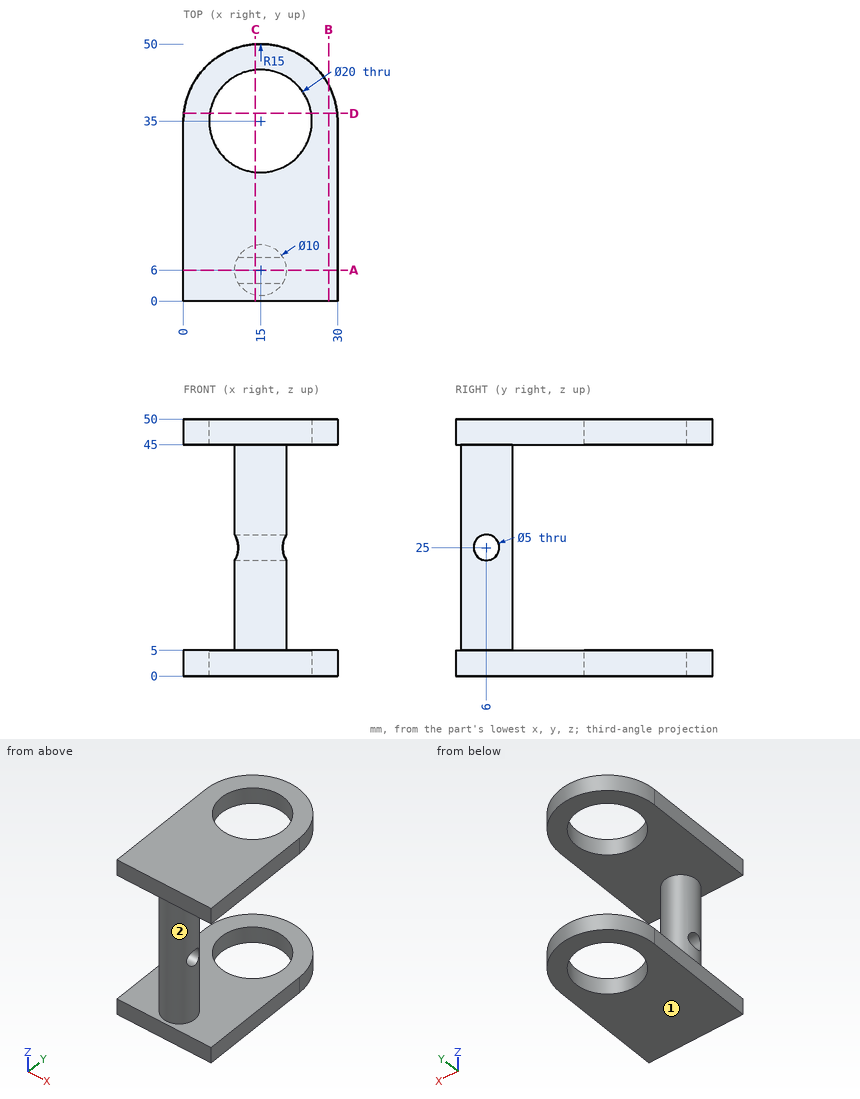
For this review, use the dimensioned drawing (mm, ordinates from the lowest corner) and the shaded views. A direction names the side the tool comes from. Give positions to 0.01 mm unless a question says otherwise; leave off trailing zeros. Order: outer loops, then holes, each group sorted by start corner. A loop starts at its lowest first (then second) coordinate and runs counter-clockwise, first axis right, second up.
1) Wall thickness on line 1 (Z direction, x = 9.75, y = 10.5); line 2 (Y direction, x = 15, z = 3.1); line 3 (Z direction, x = 15.5, y = 6): over which ranges is each line inside the solid? List them lowest first.
2) Take a section at D-D (y = 36.5). Give the boundary of the cut face in (x, z), then the cut area to 3 significant figures.
3) Take a section at B-B (x = 28.25). Give the boundary of the cut face in (y, z).
4) Take a section at A-A (y = 6). Give the boundary of the cut face in (x, z).
5) Take a section at C-C (x = 14). Give the boundary of the cut face in (y, z).
6) Insertion check: pin 1 (9 mm diameter, centred on x = 13.5, y = 12.5, fed in from -Z); pin 2 (4 mm diameter, centred on y = 6, z = 25, fed in from +X); pin 3 (6 mm diameter, centred on x = 15, z = 15.5, fed in from -Y). Each pin has a flat end and moves straight along its axis. Give the tip position at first contact, or say it passes through.
7) For the marked faces 1 and 2, list the 3-axis set-ups (+Z, -Z, +X, -X, +Y, -Y) from which the entire face can be reached by the end or side of a thin tool; tool diameter is ignored.
Derived:
1. line 1: z = 0 to 5, 45 to 50
1. line 2: y = 0 to 25, 45 to 50
1. line 3: z = 0 to 22.5, 27.5 to 50
2. outline: (0.08, 0) - (5.11, 0) - (5.11, 5) - (0.08, 5) - close; (0.08, 45) - (5.11, 45) - (5.11, 50) - (0.08, 50) - close; (24.89, 0) - (29.92, 0) - (29.92, 5) - (24.89, 5) - close; (24.89, 45) - (29.92, 45) - (29.92, 50) - (24.89, 50) - close
2. area: 101 mm2
3. outline: (0, 0) - (42.03, 0) - (42.03, 5) - (0, 5) - close; (0, 45) - (42.03, 45) - (42.03, 50) - (0, 50) - close
4. outline: (0, 0) - (30, 0) - (30, 5) - (20, 5) - (20, 22.5) - (10, 22.5) - (10, 5) - (0, 5) - close; (0, 45) - (10, 45) - (10, 27.5) - (20, 27.5) - (20, 45) - (30, 45) - (30, 50) - (0, 50) - close
5. outline: (0, 0) - (25.05, 0) - (25.05, 5) - (10.9, 5) - (10.9, 45) - (25.05, 45) - (25.05, 50) - (0, 50) - (0, 45) - (1.1, 45) - (1.1, 5) - (0, 5) - close; (44.95, 0) - (49.97, 0) - (49.97, 5) - (44.95, 5) - close; (44.95, 45) - (49.97, 45) - (49.97, 50) - (44.95, 50) - close; hole circle Ø5 at (6, 25)
6. pin 1: stops at z = 0
6. pin 2: passes through
6. pin 3: stops at y = 1
7. face 1: -Z, +X, -X, +Y, -Y
7. face 2: none
